The model under review builds one solid part; all positions refer to its coordinate system, in mm. Face numbers are marked on the shaded views. Coordinates: 2 decimals unless noted, no trailing zeros. Order: outer loops, then holes, each group sorted by start corner. A loop starts at its lowest first (then second) coordinate and runs counter-clockwise, first axis right, second up.
```python
from build123d import *

# Parameters (mm, degrees)
SKETCH1_W           = 20
SKETCH1_H           = 40
SKETCH1_R           = 5.5
BOSS_EXTRUDE1_DEPTH = 8
FILLET1_RADIUS      = 10
FILLET1_LENGTH      = 8
FILLET2_R           = 10
FILLET3_R           = 3


with BuildPart() as part:
    # Sketch1 → Boss-Extrude1 (new body)
    with BuildSketch(Plane(origin=(0, 0, 0), x_dir=(1, 0, 0), z_dir=(0, 1, 0))):
        Rectangle(SKETCH1_W, SKETCH1_H)
        with Locations(Location((0, -10, 0), (0, 0, 270))):
            Circle(SKETCH1_R, mode=Mode.SUBTRACT)
    extrude(amount=BOSS_EXTRUDE1_DEPTH)

    # Fillet1: full round fillet: the end face becomes a half cylinder, R = half its width
    fillet1_face = Plane((0, 4, 20), x_dir=(0, 1, 0), z_dir=(0, 0, 1))  # on the end face: x along it, z out of the body
    fillet1_slab = fillet1_face.offset(-FILLET1_RADIUS / 2) * Box(FILLET1_LENGTH, 2 * FILLET1_RADIUS, FILLET1_RADIUS, mode=Mode.PRIVATE)  # the body's end, R deep
    fillet1_round = Plane((0, 4, 10), x_dir=(0, 0, 1), z_dir=(0, 1, 0)) * Cylinder(FILLET1_RADIUS, FILLET1_LENGTH, mode=Mode.PRIVATE)  # its axis R under the face
    add(fillet1_slab - fillet1_round, mode=Mode.SUBTRACT)

    # Fillet2
    fillet2_edges = [part.edges().sort_by_distance(p)[0] for p in [
        (10, 4, -20),
    ]]
    fillet(fillet2_edges, radius=FILLET2_R)

    # Fillet3
    fillet3_edges = [part.edges().sort_by_distance(p)[0] for p in [
        (-10, 4, -20),
    ]]
    fillet(fillet3_edges, radius=FILLET3_R)


solid = part.part
```
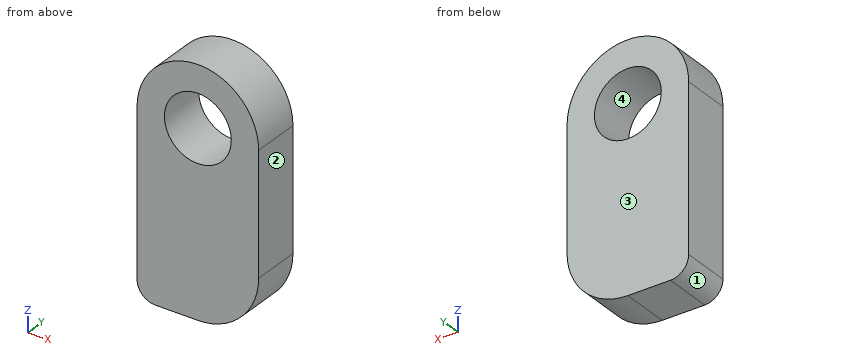
(1) We need section B-B, the plane y = 4. Write out the cut boundary in (x, z), and give its area (3 significant figures).
A:
outline: (-10, -17) arc R3 ccw to (-7, -20) - (0, -20) arc R10 ccw to (10, -10) - (10, 10) arc R10 ccw to (-10, 10) - close; hole circle Ø11 at (0, 10)
area: 639 mm2
(2) Wall thickness on probe 1 along X at (y, z) = (2.5, 10); probe 2 along Z at (x, y) = (-4.5, 6.5); probe 3 along Z at (x, y) = (-1.5, 5.25): over which ranges is each line inside the solid? List them lowest first.
A:
probe 1: x = -10 to -5.5, 5.5 to 10
probe 2: z = -20 to 6.84, 13.16 to 18.93
probe 3: z = -20 to 4.71, 15.29 to 19.89
(3) We need section A-A, the plane x = 1.25. Write out the cut boundary in (y, z).
A:
outline: (0, -19.92) - (8, -19.92) - (8, 4.64) - (0, 4.64) - close; (0, 15.36) - (8, 15.36) - (8, 19.92) - (0, 19.92) - close
(4) For pin 1 Ø10 at (x, z) = (2, -9.5) entering from -Y; pin 2 Ø1.5 at (x, y) = (4.5, 6.5) entering from +Z, all flat-tipped, find the tip position at first contact; note any pin that passes through.
A:
pin 1: stops at y = 0
pin 2: stops at z = 19.27
(5) We need section C-C, the plane z = 6. Write out the cut boundary in (x, y), and give its area (3 significant figures).
A:
outline: (-10, 0) - (-3.77, 0) - (-3.77, 8) - (-10, 8) - close; (3.77, 0) - (10, 0) - (10, 8) - (3.77, 8) - close
area: 99.6 mm2
(6) Draft analysis for pull direction X (two halves, no side actions). For the marked faces 1, 2, 3 and 4, state which applies: released by +X, released by -X, zero draft, split by the parting line, or undercut.
A:
face 1: released by -X
face 2: released by +X
face 3: zero draft
face 4: undercut
(7) We need section D-D, the plane z = -13. Write out the cut boundary in (x, y).
A:
outline: (-10, 0) - (9.54, 0) - (9.54, 8) - (-10, 8) - close
